```python
from build123d import *

# Parameters (mm, degrees)
CYLINDER001_R     = 1.5
CYLINDER001_DEPTH = 17
ARRAY_COUNT       = 8
CYLINDER_R        = 10
CYLINDER_DEPTH    = 15
CHAMFER_SIZE      = 1.5


with BuildPart() as obj1:
    # Cylinder001 → Cylinder001 (new body)
    with BuildSketch(Plane(origin=(10.5, 0, 3), x_dir=(1, 0, 0), z_dir=(0, 0, 1))):
        Circle(CYLINDER001_R)
    extrude(amount=CYLINDER001_DEPTH)

    # Array: obj1 ×8 about axis
    array_axis = Axis((0, 0, 0), (0, 0, 1))


with BuildPart() as obj1_1:
    add(obj1.part)
    for i in range(1, ARRAY_COUNT):
        add(obj1.part.rotate(array_axis, i * 360 / ARRAY_COUNT))


with BuildPart() as obj1_2:
    # Array placement: moved
    add(obj1_1.part.moved(Location((0, 0, -1))))


with BuildPart() as obj2:
    # Cylinder → Cylinder (new body)
    with BuildSketch(Plane.XY):
        Circle(CYLINDER_R)
    extrude(amount=CYLINDER_DEPTH)

    # Chamfer
    chamfer_edges = [obj2.edges().sort_by_distance(p)[0] for p in [
        (-10, 0, 15),
    ]]
    chamfer(chamfer_edges, length=CHAMFER_SIZE)

    # Cut: cut obj1
    add(obj1_2.part, mode=Mode.SUBTRACT)


solid = obj2.part
```
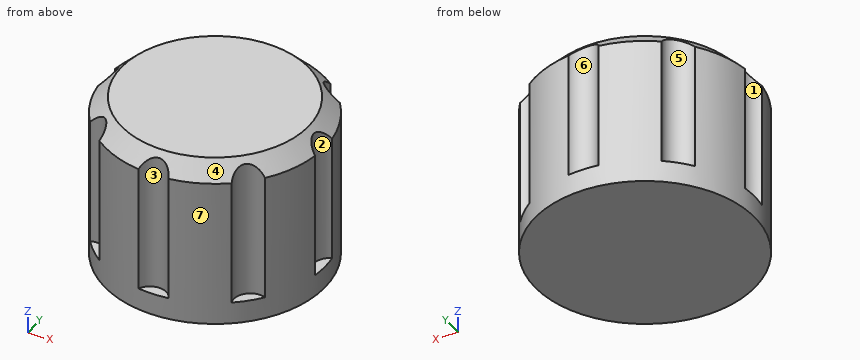
CAD build for the part. Positions are in the model's coordinates, mm. Face numbers are marked on the shaded views. A direction names the side the tool comes from. Round coordinates to 2 decimals unless told otherwise and drop trailing zeros. Write each loop counter-clockwise with the first axis right and the second up, starting at its lowest first coordinate (ties: lowest second). Pieces come first, ordered by that corner, then holes. Notation, with made-up numbers: (63, 88) -> (121, 88) arc R22 cw to (121, 119) -> close; hole circle Ø5 at (22.25, -12). An arc over 180 degrees is marked (long way). Answer in a Markdown table with one row per item. Add a question column.
Item 1: Drop flat-ended pins along their axis: pin 1 Ø8 at (y, z) = (-4, 12.5) entering from +X; pin 2 Ø0.5 at (x, y) = (-9.5, 0) entering from +Z; pin 3 Ø1.5 at (y, z) = (0, 5) entering from +X. Give the stop position or say it passes through.
Item 2: Saw through at C-C, the plane z = 12.5. Write the cut outline in (x, y).
Item 3: Drill centre lines: line 1 (Y direction, x = 9.25, z = 12); line 2 (X direction, y = 7.5, z = 3); line 3 (Z direction, x = -7, y = 6.75). Where is each one in solid material? Low to high. Write a range as from..to.
Item 4: Mould opens along Y. For the marked faces 1, 2, 3 and 4 say: pulls with the +Y half, pulls with the -Y half, needs draft (parallel to the pull), parting line crosses it, or undercut.
Item 5: Saw through at A-A, the plane y = 0. Write the cut outline in (x, z).
Item 6: Which spindle directions (+Z, -Z, +X, -X, +Y, -Y) get a long thin tool onto all of the face, cutting with end or side? Do the marked faces 5, 6 and 7. Say none if no direction does.
Findings below:
| question | item | result |
|---|---|---|
| 1 | pin 1 | stops at x = 9.9 |
| 1 | pin 2 | stops at z = 2 |
| 1 | pin 3 | stops at x = 9.2 |
| 2 | outline | (-9.9, -1.38) arc R10 ccw to (-7.98, -6.03) arc R1.5 cw to (-6.03, -7.98) arc R10 ccw to (-1.38, -9.9) arc R1.5 cw to (1.38, -9.9) arc R10 ccw to (6.03, -7.98) arc R1.5 cw to (7.98, -6.03) arc R10 ccw to (9.9, -1.38) arc R1.5 cw to (9.9, 1.38) arc R10 ccw to (7.98, 6.03) arc R1.5 cw to (6.03, 7.98) arc R10 ccw to (1.38, 9.9) arc R1.5 cw to (-1.38, 9.9) arc R10 ccw to (-6.03, 7.98) arc R1.5 cw to (-7.98, 6.03) arc R10 ccw to (-9.9, 1.38) arc R1.5 cw to start |
| 3 | line 1 | y = -3.8..-0.83, 0.83..3.8 |
| 3 | line 2 | x = -5.93..5.93 |
| 3 | line 3 | z = 0..2 |
| 4 | face 1 | undercut |
| 4 | face 2 | undercut |
| 4 | face 3 | pulls with the -Y half |
| 4 | face 4 | parting line crosses it |
| 5 | outline | (-10, 0) -> (10, 0) -> (10, 2) -> (9, 2) -> (9, 14.5) -> (8.5, 15) -> (-8.5, 15) -> (-9, 14.5) -> (-9, 2) -> (-10, 2) -> close |
| 6 | face 5 | +Z |
| 6 | face 6 | +Z, +Y |
| 6 | face 7 | +Z, -Z |
